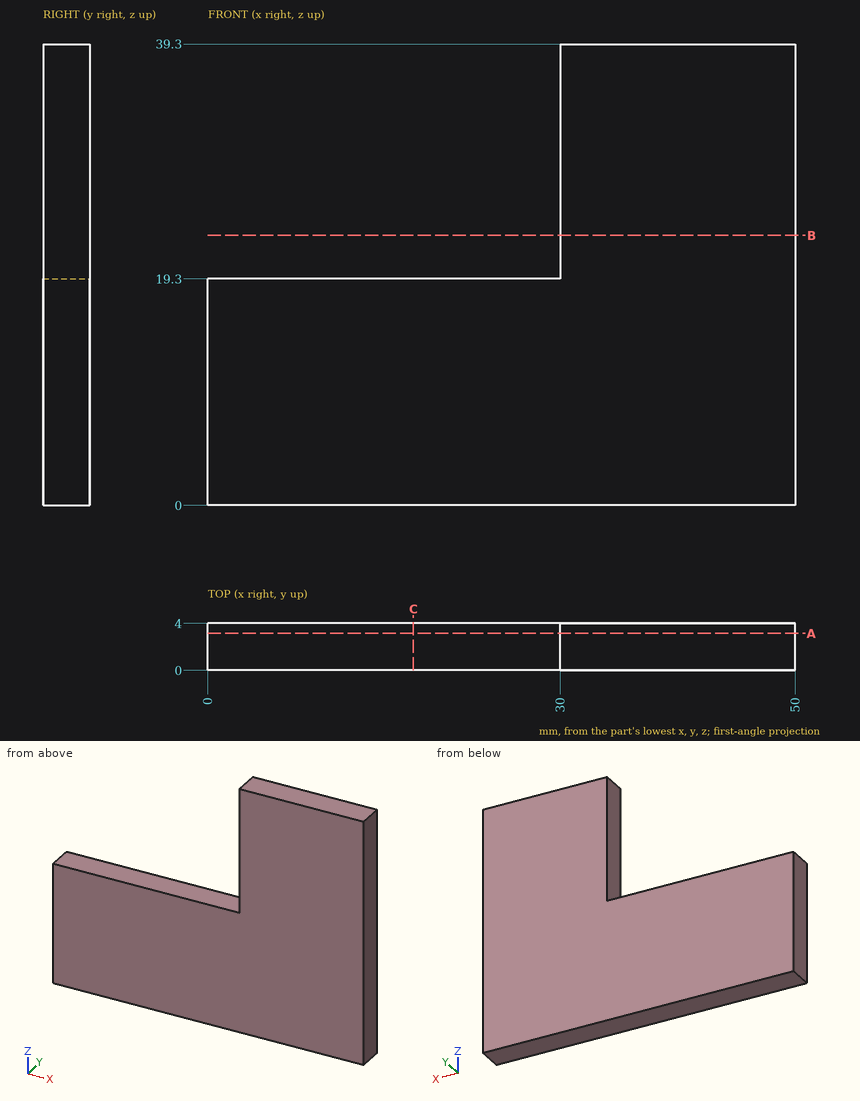
Drawing for the job (mm, zero at the part's lowest x, y, z). Give positions to 0.01 mm unless a question says otherwise; leave off trailing zeros. Loops run counter-clockwise (first coordinate to the right, second up) from the corner with the lowest first, then second, coordinate; pieces in that order, holes last.
(1) Drill centre lines: line 1 along X through (y, z) = (3.85, 31.5); line 2 along Z through (x, y) = (29, 3.7). Where is each one in solid material? Low to high.
Return value:
line 1: x = 30 to 50
line 2: z = 0 to 19.3
(2) Pin check, flat tip, straight feed: pin 1 (2 mm diameter, centred on y = 2, z = 29.5, fed in from -X). Stop position of the tip, or through.
Return value:
pin 1: stops at x = 30
(3) Band-saw the part on C-C (x = 17.5). Write the cut outline in (y, z), and give its area (3 significant figures).
Return value:
outline: (0, 0) - (4, 0) - (4, 19.3) - (0, 19.3) - close
area: 77.2 mm2
(4) Band-saw the part on A-A (y = 3.15). Write the cut outline in (x, z).
Return value:
outline: (0, 0) - (50, 0) - (50, 39.3) - (30, 39.3) - (30, 19.3) - (0, 19.3) - close
(5) Band-saw the part on B-B (z = 23). Write the cut outline in (x, y).
Return value:
outline: (30, 0) - (50, 0) - (50, 4) - (30, 4) - close
